```python
from build123d import *

# Parameters (mm, degrees)
F0_W         = 9.525
F0_H         = 9.525
F1_DEPTH     = 2.286
F2_T1_DEPTH  = 21.3619144247
F3_W         = 2.9083
F3_H         = 9.525
F3_W_2       = 6.8834
F4_DEPTH     = 1.905
F5_R         = 1.6556676611
F6_W         = 12.7
F6_H         = 1.27
F7_DEPTH     = 3.429
F8_SIZE2     = 8.7232408068
F8_SIZE      = 3.175
F9_T4_DEPTH  = 12.7
F9_T9_DEPTH  = 12.7
F10_T1_DEPTH = 21.1289299719


# Not quite as in the source:
# - a fillet or chamfer that OpenCascade refuses, or shapes differently, is made with other operations: its cross-section is extruded or revolved along the edge and cut away or added


with BuildPart() as f1:
    # F0 (on Top) → F1 (new body)
    with BuildSketch(Plane.XY):
        Rectangle(F0_W, F0_H)
    extrude(amount=F1_DEPTH)

    # F2: chamfer of 1.3208 x 2.2876927066 on 2 edges, made by hand

    # F2_s2 → F2_t1 (cut)
    with BuildSketch(Plane.XZ.offset(-10.6809572123)):
        Polygon((-4.7625, -0.0016927066), (-3.4417, 2.286), (-4.7625, 2.286), align=None)
        Polygon((4.7625, -0.0016927066), (3.4417, 2.286), (4.7625, 2.286), align=None)
    extrude(amount=F2_T1_DEPTH, mode=Mode.SUBTRACT)

    # F3 (on face) → F4 (join)
    with BuildSketch(Plane.XY.offset(2.286)):
        with Locations((4.89585, 0)):
            Rectangle(F3_W, F3_H)
        Rectangle(F3_W_2, F3_H)
        with Locations((-4.89585, 0)):
            Rectangle(F3_W, F3_H)
    extrude(amount=F4_DEPTH)

    # F5
    f5_edges = [f1.edges().sort_by_distance(p)[0] for p in [
        (0, 4.7625, 4.191),
        (0, -4.7625, 4.191),
    ]]
    fillet(f5_edges, radius=F5_R)

    # F6 (on face) → F7 (join)
    with BuildSketch(Plane.XY.offset(4.191)):
        Rectangle(F6_W, F6_H)
    extrude(amount=F7_DEPTH)

    # F8
    f8_edges = [f1.edges().sort_by_distance(p)[0] for p in [
        (-6.35, 0, 7.62),
    ]]
    f8_side = f1.faces().sort_by_distance((-6.35, 0, 3.751025))[0]
    chamfer(f8_edges, length=F8_SIZE, length2=F8_SIZE2, reference=f8_side)

    # F9: fillet of radius 2.8207671263 on 2 edges, made by hand


with BuildPart() as f9_tool2:
    # F9_s3 → F9_t4 (new body)
    with BuildSketch(Plane.YZ.offset(-6.35)):
        with BuildLine():
            ThreePointArc((-0.635, 6.9981468006), (-1.3849039981, 5.0828783899), (-3.235890411, 4.1859623453))
            Line((-3.235890411, 4.1859623453), (-3.2139027394, 3.9047438998))
            ThreePointArc((-3.2139027394, 3.9047438998), (-3.1068323389, 3.9089232874), (-0.635, 3.9089232874))
            Line((-0.635, 3.9089232874), (-0.3529232874, 4.191))
            Line((-0.3529232874, 4.191), (-0.3529232874, 6.9981468006))
            Line((-0.3529232874, 6.9981468006), (-0.635, 6.9981468006))
        make_face()
    extrude(amount=F9_T4_DEPTH)

    split(bisect_by=Plane(origin=(-2.1714043556, 0, 5.9658844356), x_dir=(0, 1, 0), z_dir=(0.3420201433, 0, -0.9396926208)), keep=Keep.TOP)


with BuildPart() as f1_1:
    add(f1.part)

    # F9_t1: union F9_tool2
    add(f9_tool2.part)


with BuildPart() as f9_tool7:
    # F9_s8 → F9_t9 (new body)
    with BuildSketch(Plane.YZ.offset(6.35)):
        with BuildLine():
            ThreePointArc((0.635, 6.9981468006), (1.3849039981, 5.0828783899), (3.235890411, 4.1859623453))
            Line((3.235890411, 4.1859623453), (3.2139027394, 3.9047438998))
            ThreePointArc((3.2139027394, 3.9047438998), (3.1068323389, 3.9089232874), (0.635, 3.9089232874))
            Line((0.635, 3.9089232874), (0.3529232874, 4.191))
            Line((0.3529232874, 4.191), (0.3529232874, 6.9981468006))
            Line((0.3529232874, 6.9981468006), (0.635, 6.9981468006))
        make_face()
    extrude(amount=-F9_T9_DEPTH)

    split(bisect_by=Plane(origin=(-2.1714043556, 0, 5.9658844356), x_dir=(0, 1, 0), z_dir=(0.3420201433, 0, -0.9396926208)), keep=Keep.TOP)


with BuildPart() as f1_2:
    add(f1_1.part)

    # F9_t6: union F9_tool7
    add(f9_tool7.part)

    # F10: fillet of radius 5.08 on 1 edges, made by hand

    # F10_s2 → F10_t1 (cut)
    with BuildSketch(Plane.XZ.offset(-10.564464986)):
        with BuildLine():
            ThreePointArc((-6.35, 2.286), (-5.1772680397, 4.3020632997), (-3.2272380907, 5.5815923837))
            Line((-3.2272380907, 5.5815923837), (-3.2619873372, 5.677065154))
            Line((-3.2619873372, 5.677065154), (-6.3847492466, 4.5404727703))
            Line((-6.3847492466, 4.5404727703), (-6.4516, 4.445))
            ThreePointArc((-6.4516, 4.445), (-6.4516, 3.3655), (-6.4472044847, 2.3155609226))
            Line((-6.4472044847, 2.3155609226), (-6.35, 2.286))
        make_face()
    extrude(amount=F10_T1_DEPTH, mode=Mode.SUBTRACT)


solid = f1_2.part
```
Check sheet for the modelled part. Datum: model origin and axes. Units: mm. A direction names the side the tool comes from. Round coordinates to 2 decimals unless told otherwise and drop trailing zeros. Loops run counter-clockwise (first coordinate to the right, second up) from the corner with the lowest first, then second, coordinate; pieces in that order, holes last. Notation, with made-up numbers: (67, -6) - (111, -6) arc R19 ccw to (111, 31) - close; hole circle Ø9 at (26.5, 72.5). An arc over 180 degrees is marked (long way). Write item = value, one per line. Start each with the question number.
Q1. Section check C-C (x = -4.25). Record the boundary of the cut face in (y, z), plus the area to 3 significant figures.
Q2. Access from +Z, -Z, +X, -X, +Y, -Y to the whole of each face (thin tool, end or side, straight path). Record for faces 4 (the face through (-5, 0, 2.286)), 5 (the face through (5, 0, 2.286)), 6 (the face through (-5.537, 0.067, 3.878)).
Q3. Section check D-D (z = 6.5). Record the boundary of the cut face in (x, y) (3 decimals), plus the area to 3 significant figures.
Q4. Depth check by flat-ended pin: P1, Ø0.5, axis at x = 2.5, z = 7.5, coming from the -Y side (3 decimals); P2, Ø0.5, axis at x = 3.5, z = 7, coming from the +Y side; P3, Ø4, axis at x = 0, y = 3, coming from the +Z side. Enter the tip coordinate at first touch or a pass-through.
Q5. Section check B-B (y = -3.5). Record the boundary of the cut face in (x, z).
Q6. Release check for a two-part mould opening along Z. For faces 1 (the face through (4, 0, 7.62)), 2 (the face through (4.11, 0.07, 1.13)), 3 (the face through (0, 0, 0)) record: pulls with the +Z half, pulls with the -Z half, needs draft (parallel to the pull), parting line crosses it, or undercut.
Q7. Thickness scan on L1, parallel to Z at x = -4, y = -1.5; L2, parallel to Z at x = -4, y = -0.25; L3, parallel to Y at x = 2.25, z = 5.75. Record the ranges inside material, lowest first.
Derived:
q1.outline = (-4.76, 0) - (4.76, 0) - (4.76, 0.89) - (-4.76, 0.89) - close; (-4.76, 2.29) - (4.76, 2.29) - (4.76, 2.54) arc R1.66 ccw to (3.24, 4.19) arc R2.82 cw to (1.39, 5.07) - (-1.39, 5.07) arc R2.82 cw to (-3.24, 4.19) arc R1.66 ccw to (-4.76, 2.54) - close
q1.area = 29.0 mm^2
q2.face_4 = -X, +Y, -Y
q2.face_5 = +X, +Y, -Y
q2.face_6 = +Z, -X, +Y, -Y
q3.outline = (-0.704, -0.679) - (6.35, -0.679) - (6.35, 0.679) - (-0.704, 0.679) - close
q3.area = 9.58 mm^2
q4.P1 = -0.635
q4.P2 = 0.65
q4.P3 = 5.61
q5.outline = (-6.35, 2.29) - (-3.44, 2.29) - (-4.76, 0) - (4.76, 0) - (3.44, 2.29) - (6.35, 2.29) - (6.35, 4.14) - (-5.32, 4.14) arc R5.08 ccw to start
q6.face_1 = pulls with the +Z half
q6.face_2 = undercut
q6.face_3 = pulls with the -Z half
q7.L1 = 0 to 1.32, 2.29 to 4.97
q7.L2 = 0 to 1.32, 2.29 to 5.22
q7.L3 = -0.93 to 0.93
